Design review of the part built by this model. Coordinates are the model's own, in mm. A direction names the side the tool comes from. Give positions to 0.01 mm unless a question says otherwise; leave off trailing zeros. Order: outer loops, then holes, each group sorted by start corner. A loop starts at its lowest first (then second) coordinate and runs counter-clockwise, first axis right, second up. Notation, with made-up numbers: M -24,26.25 L 6,26.25 A11 cw 6,30.25 Z; hole C 7,21.5 d6. An arc over 180 degrees is marked long. Answer as a JSON object with one key per item and string values.
from build123d import *

# Parameters (mm, degrees)
BOSS_EXTRUDE2_DEPTH      = 25.4
BOSS_EXTRUDE2_DEPTH_BACK = 19.05
SKETCH3_R                = 3.175
CUT_EXTRUDE5_DEPTH       = 26.793821935
CUT_EXTRUDE5_DEPTH_BACK  = 26.793821935
SKETCH10_W               = 2.38125
SKETCH10_H               = 1.422321225
CHAMFER1_SIZE            = 0.3175


with BuildPart() as part:
    # Sketch3 → Boss-Extrude2 (new, two sides: drawn at the far end of the back side and taken through both)
    with BuildSketch(Plane.XY.offset(-BOSS_EXTRUDE2_DEPTH_BACK)):
        Circle(SKETCH3_R)
    extrude(amount=BOSS_EXTRUDE2_DEPTH + BOSS_EXTRUDE2_DEPTH_BACK)

    # Sketch10 → Cut-Extrude5 (cut, two sides: drawn at the far end of the back side and taken through both)
    with BuildSketch(Plane.XY.offset(-CUT_EXTRUDE5_DEPTH_BACK)):
        with Locations((0, 2.463839388)):
            Rectangle(SKETCH10_W, SKETCH10_H)
    extrude(amount=CUT_EXTRUDE5_DEPTH + CUT_EXTRUDE5_DEPTH_BACK, mode=Mode.SUBTRACT)

    # Chamfer1
    chamfer1_edges = [part.edges().sort_by_distance(p)[0] for p in [
        (0, -3.175, -19.05),
        (0, -3.175, 25.4),
    ]]
    chamfer(chamfer1_edges, length=CHAMFER1_SIZE)


solid = part.part
(1) To check wall thickness, follow L1, parallel to X at y = 2.5, z = -9; L2, parallel to X at y = 1.5, z = 15; L3, parallel to X at y = -2, z = -17. State the ranges of each line that lie inside material, in increasing order. Write a range as from..to.
Checked values:
{"L1": "x = -1.96..-1.19, 1.19..1.96", "L2": "x = -2.8..2.8", "L3": "x = -2.47..2.47"}
(2) Draft analysis for pull direction X (two halves, no side actions). For faces 3 (the flat face through (-1.191, 2, 3)), 4 (the flat face through (0, 0, 25.4)), 5 (the conical face through (-0.115, -2.977, -18.929)), state which applies: +X half, -X half, draft (parallel to the pull), parting line (faces both ways), or undercut.
Checked values:
{"face 3": "undercut", "face 4": "draft", "face 5": "parting line"}
(3) Tool access review of faces 1 (the conical face through (0.115, -2.977, 25.279)), 2 (the flat face through (1.191, 2, 3)): name each direction out of +Z, -Z, +X, -X, +Y, -Y from which nothing blocks a thin tool from reaching the whole face with its end or side.
Checked values:
{"face 1": "+Z", "face 2": "+Z, -Z, +Y"}
(4) Insertion check: pin 1 (2 mm diameter, centred on y = 2, z = -2, fed in from -X); pin 2 (1 mm diameter, centred on y = 2.5, z = -5.5, fed in from -X); pin 3 (0.7 mm diameter, centred on x = -0.5, z = 1, fed in from +Y). Each pin has a flat end and moves straight along its axis. Give the tip position at first contact, or say it passes through.
Checked values:
{"pin 1": "stops at x = -3.01", "pin 2": "stops at x = -2.47", "pin 3": "stops at y = 1.75"}
(5) We need section B-B (z = -16). Write out the cut boundary in (x, y) (3 decimals), plus the area to 3 significant figures.
Checked values:
{"outline": "M -1.191,1.753 L -1.191,2.943 A3.175 ccw long 1.191,2.943 L 1.191,1.753 Z", "area": "28.5 mm^2"}
